from build123d import *

# Parameters (mm, degrees)
CUT_EXTRUDE_1_DEPTH = 0.5
FILLET_1_R          = 1


with BuildPart() as part:
    # 草图1 → 旋转1 (revolve)
    with BuildSketch(Plane.XY, mode=Mode.PRIVATE) as revolve_1_sk:
        Polygon((0, 0), (0, 1.9), (1.6, 1.9), (1.6, 1.1), (6.5, 1.1), (7.6, 0), align=None)
    revolve(revolve_1_sk.sketch.rotate(Axis((-6.976540153, 0, 0), (1, 0, 0)), 90), axis=Axis((-6.976540153, 0, 0), (1, 0, 0)))

    # 草图2 → 切除-拉伸1 (cut)
    with BuildSketch(Plane.ZY):
        Polygon((-0.3, 0.3), (-1, 0.3), (-1, -0.3), (-0.3, -0.3), (-0.3, -1), (0.3, -1), (0.3, -0.3), (1, -0.3), (1, 0.3), (0.3, 0.3), (0.3, 1), (-0.3, 1), align=None)
    extrude(amount=-CUT_EXTRUDE_1_DEPTH, mode=Mode.SUBTRACT)

    # 圆角1
    # the kernel refuses this fillet: 1 mm, written as the material it takes off along each edge
    with BuildSketch(Plane(origin=(0, 0, 0), x_dir=(0, 0, 1), z_dir=(0, 1, 0))) as fillet_1_piece_1:
        with BuildLine():
            CenterArc((1.9 - FILLET_1_R, FILLET_1_R), FILLET_1_R, 270, 90)
            Line((1.9, FILLET_1_R), (1.9, 0))
            Line((1.9, 0), (1.9 - FILLET_1_R, 0))
        make_face()
    revolve(axis=Axis((0, 0, 0), (1, 0, 0)), mode=Mode.SUBTRACT)


solid = part.part
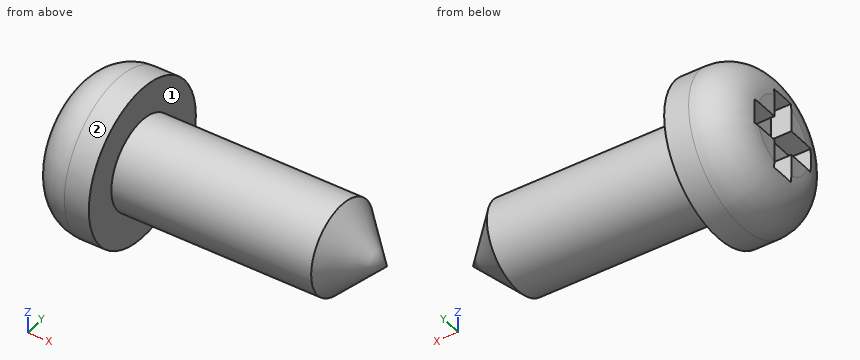
Read the model definition and answer for the solid it produces. Units are mm, in the model's axes. Face numbers are marked on the shaded views. A direction names the side the tool comes from. Coordinates: 2 decimals unless noted, no trailing zeros. Write each loop counter-clockwise with the first axis right and the second up, starting at its lowest first coordinate (ties: lowest second). Pieces come first, ordered by that corner, then holes. Notation, with made-up numbers: (26, 73) -> (77, 73) arc R27 ccw to (77, 102) -> close; hole circle Ø1 at (28.25, 49). An arc over 180 degrees is marked (long way). Return JSON: item names as keys, results as strings.
(1) Each of these flat-tipped pins is pushed along its axis until it touches: P1, Ø1.5, axis at x = 5.5, y = -0.5, coming from the +Z side; P2, Ø0.6, axis at x = 0, z = -0.5, coming from the +Y side; P3, Ø0.6, axis at x = 0, y = 0.5, coming from the -Z side. Where does it stop, or does it pass through?
Answers below:
{"P1": "z = 1.1", "P2": "y = 1.55", "P3": "z = -1.55"}
(2) The part is cut by section A-A on x = 1.5. Give the vertices of the cut face in (y, z).
Answers below:
{"outline": "circle Ø3.8 at (0, 0)"}
(3) Which of the six approach directions +Z, -Z, +X, -X, +Y, -Y give full straight-line access (tool end or side, diameter ignored) to the marked faces 1 and 2?
Answers below:
{"face 1": "+X", "face 2": "+X, -X"}
(4) Consider line 1 along X through (y, z) = (-1.7, -0.1); line 2 along Y through (x, z) = (4.75, 0.3); line 3 along Y through (x, z) = (7.25, -0.15). Determine where each line is inside the solid, lowest interval first. Write a range as from..to.
Answers below:
{"line 1": "0.4..1.6", "line 2": "-1.06..1.06", "line 3": "-0.32..0.32"}
